The listing builds one solid part. Answer for the finished solid, in the listing's coordinates (mm). A direction names the side the tool comes from. Give positions to 0.01 mm unless a question says otherwise; leave off trailing zeros. Loops run counter-clockwise (first coordinate to the right, second up) from the corner with the lowest first, then second, coordinate; pieces in that order, holes last. Notation, with made-up numbers: M 19,3.25 L 39,3.25 A36 cw 39,40.25 Z; hole C 55,42.25 d11. An arc over 180 degrees is marked long. Return JSON: item names as keys, results as strings.
from build123d import *

# Parameters (mm, degrees)
BOSS_EXTRUDE1_DEPTH            = 5
BOSS_EXTRUDE1_DEPTH_BACK       = 5
FILLET1_R                      = 1
F_4_0MM_DOWEL_HOLE1_AT_2_COUNT = 2
F_4_0MM_DOWEL_HOLE1_AT_2_PITCH = 10


with BuildPart() as part:
    # Sketch1 → Boss-Extrude1 (new body, two sides)
    with BuildSketch(Plane.XY) as boss_extrude1_sk:
        with BuildLine():
            Line((0, 0), (40, 0))
            Line((40, 0), (40, 8))
            ThreePointArc((40, 8), (29.039542787, 18.960457213), (18.079085573, 8))
            Line((18.079085573, 8), (0, 8))
            Line((0, 8), (0, 5))
            Line((0, 5), (21.079085573, 5))
            Line((21.079085573, 5), (21.079085573, 7.695472827))
            ThreePointArc((21.079085573, 7.695472827), (29.562443146, 14.553574165), (37, 6.57337005))
            Line((37, 6.57337005), (37, 3))
            Line((37, 3), (0, 3))
            Line((0, 3), (0, 0))
        make_face()
    extrude(amount=BOSS_EXTRUDE1_DEPTH)
    extrude(boss_extrude1_sk.sketch, amount=-BOSS_EXTRUDE1_DEPTH_BACK)

    # Fillet1
    fillet1_edges = [part.edges().sort_by_distance(p)[0] for p in [
        (0, 6.5, -5),
        (0, 1.5, 5),
        (0, 6.5, 5),
        (0, 1.5, -5),
    ]]
    fillet(fillet1_edges, radius=FILLET1_R)

    # Sketch5 → 4.0mm Dowel Hole1 (revolve, cut)
    with BuildSketch(Plane(origin=(8, 8, 0), x_dir=(0, 0, 1), z_dir=(1, 0, 0))):
        Polygon((0, 0), (0, 8), (2, 8), (2, 0.025), (2.025, 0), align=None)
    f_4_0mm_dowel_hole1 = revolve(axis=Axis((8, 14.35, 0), (0, -1, 0)), mode=Mode.SUBTRACT)

    # 4.0mm Dowel Hole1 at 2: 4.0mm Dowel Hole1 ×2
    with Locations(*[(i * F_4_0MM_DOWEL_HOLE1_AT_2_PITCH, 0, 0) for i in range(1, F_4_0MM_DOWEL_HOLE1_AT_2_COUNT)]):
        add(f_4_0mm_dowel_hole1, mode=Mode.SUBTRACT)


solid = part.part
(1) The part is cut by section D-D (y = 1.5). Determine the outline of the cut face in (x, z).
Values follow:
{"outline": "M 0,-4 A1 ccw 1,-5 L 40,-5 L 40,5 L 1,5 A1 ccw 0,4 Z; hole C 8,0 d4; hole C 18,0 d4"}
(2) The part is cut by section B-B (y = 5.5). Determine the outline of the cut face in (x, z), and give its area (3 significant figures).
Values follow:
{"outline": "M 0,-4 A1 ccw 1,-5 L 21.08,-5 L 21.08,5 L 1,5 A1 ccw 0,4 Z; M 37,-5 L 40,-5 L 40,5 L 37,5 Z; hole C 8,0 d4; hole C 18,0 d4", "area": "215 mm²"}
(3) Straight lines are drawn through the part: line 1 along X through (y, z) = (6.6, 0); line 2 along Z through (x, y) = (18, 2.4); line 3 along X through (y, z) = (1.75, 1.5). For each, find the intervals that lie inside material, in ascending order.
Values follow:
{"line 1": "0 to 6, 10 to 16, 20 to 21.08, 37 to 40", "line 2": "-5 to -2, 2 to 5", "line 3": "0 to 6.68, 9.32 to 16.68, 19.32 to 40"}
(4) The part is cut by section A-A (z = 0). Give the number of separate pieces and of enclosed holes in the cut face, and give its area (3 significant figures).
Values follow:
{"separate pieces": "5", "enclosed holes": "0", "area": "261 mm²"}
(5) Given pin 1 (5 mm diameter, centred on x = 18, z = 0, fed in from -Y); pin 2 (3 mm diameter, centred on x = 19.5, z = 1, fed in from +Y); pin 3 (2.5 mm diameter, centred on x = 8, z = 0, fed in from +Y); pin 4 (5 mm diameter, centred on x = 13, z = -2, fed in from +Y), each flat-ended and moving along its own axis, determine where each tip first touches the part or whether it passes through.
Values follow:
{"pin 1": "y = 0", "pin 2": "y = 15.45", "pin 3": "through", "pin 4": "y = 8"}
(6) A tool of negligible diameter and unlimited length cuts with its end or side. For faces 1 (the flat face through (20, 8, -5)), 2 (the cylindrical face through (16, 2, 0)), 3 (the flat face through (37, 5, 0)), 4 (the flat face through (19, 3, 2)), 5 (the cylindrical face through (0.285, 1.479, 4.699)), from which of +Z, -Z, +X, -X, +Y, -Y can it reach the whole face along a straight path? Write none if from no direction.
Values follow:
{"face 1": "-Z, +X, -X, +Y, -Y", "face 2": "-Y", "face 3": "+Z, -Z", "face 4": "+Z, -Z, -X", "face 5": "+Z, -X, +Y, -Y"}
(7) The part is cut by section C-C (x = 8). Determine the outline of the cut face in (y, z) (3 decimals), and give its area (3 significant figures).
Values follow:
{"outline": "M 0,-5 L 3,-5 L 3,-2 L 0,-2 Z; M 0,2 L 3,2 L 3,5 L 0,5 Z; M 5,-5 L 8,-5 L 8,-2.025 L 7.975,-2 L 5,-2 Z; M 5,2 L 7.975,2 L 8,2.025 L 8,5 L 5,5 Z", "area": "36.0 mm²"}
(8) Determine the mould class of faces 6 (the cylindrical face through (6, 2, 0)), 7 (the cylindrical face through (6, 7, 0)), 8 (the flat face through (40, 4, 0)), 9 (the flat face through (20, 8, 5)) for opening direction Z: released by +Z, released by -Z, zero draft, split by the parting line, or undercut.
Values follow:
{"face 6": "undercut", "face 7": "undercut", "face 8": "zero draft", "face 9": "released by +Z"}
